```python
from build123d import *

# Parameters (mm, degrees)
F0_W     = 152.4
F0_H     = 50.8
F1_DEPTH = 76.2
F2_W     = 131.459884
F2_H     = 25.4
F3_DEPTH = 25.4
F4_W     = 131.459884
F4_H     = 25.4
F5_DEPTH = 25.4
F7_DEPTH = 25.4


with BuildPart() as f1:
    # F0 (on Front) → F1 (new body)
    with BuildSketch(Plane.XZ):
        with Locations((135.731251, 25.4)):
            Rectangle(F0_W, F0_H)
    extrude(amount=F1_DEPTH)

    # F2 (on face) → F3 (cut)
    with BuildSketch(Plane.XY.offset(50.8)):
        with Locations((146.201309, -63.5)):
            Rectangle(F2_W, F2_H)
    extrude(amount=-F3_DEPTH, mode=Mode.SUBTRACT)

    # F4 (on face) → F5 (cut)
    with BuildSketch(Plane.XY.offset(50.8)):
        with Locations((146.201309, -12.7)):
            Rectangle(F4_W, F4_H)
    extrude(amount=-F5_DEPTH, mode=Mode.SUBTRACT)

    # F6 (on face) → F7 (cut)
    with BuildSketch(Plane.XZ.offset(50.8)):
        Polygon((211.931251, 50.8), (80.471367, 50.8), (211.931251, 25.4), align=None)
    extrude(amount=-F7_DEPTH, mode=Mode.SUBTRACT)


solid = f1.part
```
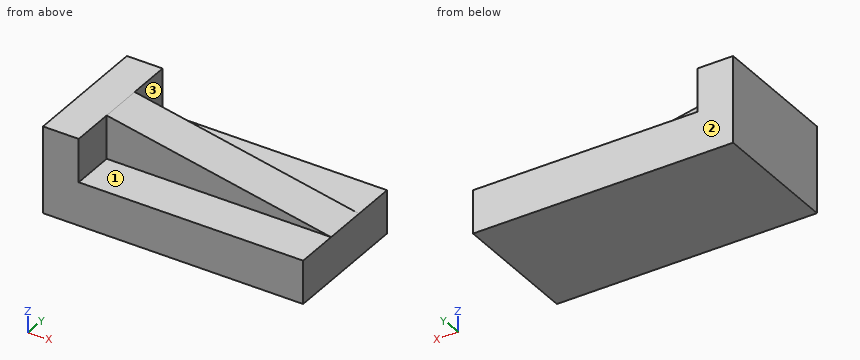
Read the model definition and answer for the solid it produces. Units are mm, in the model's axes. Face numbers are marked on the shaded views. A direction names the side the tool comes from. Give positions to 0.01 mm unless a question says otherwise; leave off trailing zeros. Loops run counter-clockwise (first coordinate to the right, second up) from the corner with the lowest first, then second, coordinate; pieces in that order, holes last.
Item 1: The part is cut by section A-A (y = -67). Write down the section's boundary in (x, z), and give its area (3 significant figures).
Item 2: The part is cut by section B-B (x = 202). Write down the section's boundary in (y, z).
Item 3: For the marked faces 1, 2 and 3, determine the directions among +Z, -Z, +X, -X, +Y, -Y from which every point of the face is accessible in a straight line to the end or side of a thin tool.
Item 4: The part is cut by section D-D (y = -44). Write down the section's boundary in (x, z).
Item 5: Each of these flat-tipped pins is pushed along its axis until it touches: pin 1 Ø7.5 at (x, z) = (116, 37) entering from +Y; pin 2 Ø6 at (x, z) = (108.5, 43.5) entering from -Y; pin 3 Ø20.5 at (x, y) = (115, -62.5) entering from +Z; pin 4 Ø4 at (x, y) = (105, -25) entering from -Z. Where does it stop, or does it pass through?
Item 6: The part is cut by section C-C (z = 35.5). Write down the section's boundary in (x, y).
Item 7: Find the intervals of material crossed by line 1 along Z through (x, y) = (103, -20.5); line 2 along Y through (x, z) = (87, 29.5); line 3 along X through (y, z) = (-11, 41), in increasing order.
Taken from the geometry:
1. outline: (59.53, 0) - (211.93, 0) - (211.93, 25.4) - (80.47, 25.4) - (80.47, 50.8) - (59.53, 50.8) - close
1. area: 4,400 mm2
2. outline: (-76.2, 0) - (0, 0) - (0, 25.4) - (-25.4, 25.4) - (-25.4, 27.32) - (-50.8, 27.32) - (-50.8, 25.4) - (-76.2, 25.4) - close
3. face 1: +Z, +X, -Y
3. face 2: +Z, -Z, +X, -X, +Y
3. face 3: +Z, +X, +Y
4. outline: (59.53, 0) - (211.93, 0) - (211.93, 25.4) - (80.47, 50.8) - (59.53, 50.8) - close
5. pin 1: stops at y = -25.4
5. pin 2: stops at y = -50.8
5. pin 3: stops at z = 25.4
5. pin 4: stops at z = 0
6. outline: (59.53, -76.2) - (80.47, -76.2) - (80.47, -50.8) - (159.66, -50.8) - (159.66, -25.4) - (80.47, -25.4) - (80.47, 0) - (59.53, 0) - close
7. line 1: z = 0 to 25.4
7. line 2: y = -50.8 to -25.4
7. line 3: x = 59.53 to 80.47
